from build123d import *

# Parameters (mm, degrees)
FILLET1_R       = 0.2
FILLET2_R       = 0.25
HEX_2_DEPTH     = 2.5
THDSCHPAT_COUNT = 17
THDSCHPAT_PITCH = 0.8


with BuildPart() as part:
    # BodySke → Base-Revolve (revolve)
    with BuildSketch(Plane.XY):
        Polygon((0, 0), (0, 4.25), (5, 4.25), (5, 2.5), (20.555, 2.5), (21, 2.055), (21, 0), align=None)
    revolve(axis=Axis((-31.75, 0, 0), (1, 0, 0)))

    # Fillet1
    fillet1_edges = [part.edges().sort_by_distance(p)[0] for p in [
        (5, -2.5, 0),
    ]]
    fillet(fillet1_edges, radius=FILLET1_R)

    # Fillet2
    fillet2_edges = [part.edges().sort_by_distance(p)[0] for p in [
        (0, -4.25, 0),
    ]]
    fillet(fillet2_edges, radius=FILLET2_R)

    # Sketch2 → Hex-PreBroach (revolve, cut)
    with BuildSketch(Plane.XY):
        Polygon((0, 2.042), (2.5, 2.042), (3.67894925, 0), (0, 0), align=None)
    revolve(axis=Axis((0, 0, 0), (1, 0, 0)), mode=Mode.SUBTRACT)

    # Sketch3 → Hex 2 (cut)
    with BuildSketch(Plane(origin=(0, 0, 0), x_dir=(0, 0.5, 0.866025404), z_dir=(-1, 0, 0))):
        Polygon((1.17894925, 2.042), (-1.17894925, 2.042), (-2.357898499, 0), (-1.17894925, -2.042), (1.17894925, -2.042), (2.357898499, 0), align=None)
    extrude(amount=-HEX_2_DEPTH, mode=Mode.SUBTRACT)

    # ThdSchSke → ThreadSchematic (revolve, cut)
    with BuildSketch(Plane.XY):
        Polygon((7.4, -2.055), (7.088407645, -2.5), (7.088407645, -3.125), (7.711592355, -3.125), (7.711592355, -2.5), align=None)
    threadschematic = revolve(axis=Axis((-3.175, 0, 0), (1, 0, 0)), mode=Mode.SUBTRACT)

    # ThdSchPat: ThreadSchematic ×17
    with Locations(*[(i * THDSCHPAT_PITCH, 0, 0) for i in range(1, THDSCHPAT_COUNT)]):
        add(threadschematic, mode=Mode.SUBTRACT)


solid = part.part
Verification items for the finished model (mm, model axes). A direction names the side the tool comes from. Round coordinates to 2 decimals unless told otherwise and drop trailing zeros. Write item = value, one per line.
Q1. Tool access check on faces 1 (the cylindrical face through (2.658, 2.285, 3.584)), 2 (the cylindrical face through (6.16, -0.54, -2.44)). Record the directions out of +Z, -Z, +X, -X, +Y, -Y that give a thin tool (end or side, any length) a straight path to the whole face; none if there is none.
Here are the results:
face_1 = +X, -X
face_2 = +X
Q2. Material ranges on L1, parallel to X at y = 1.75, z = 2.25; L2, parallel to Z at x = 2, y = -1; L3, parallel to Z at x = 4, y = -2.5, recorded low to high.
Here are the results:
L1 = 0 to 5
L2 = -4.13 to -2.04, 2.04 to 4.13
L3 = -3.44 to 3.44
Q3. Depth check by flat-ended pin: pin 1 (4 mm diameter, centred on x = 7.5, z = 2, fed in from -Y); pin 2 (0.5 mm diameter, centred on y = -2, z = 0, fed in from -X); pin 3 (0.5 mm diameter, centred on y = 0.5, z = -1.5, fed in from -X). Enter the tip coordinate at first touch or a pass-through.
Here are the results:
pin_1 = -2.5
pin_2 = 2.5
pin_3 = 2.62
